Design review of the part built by this model. Coordinates are the model's own, in mm. A direction names the side the tool comes from. Give positions to 0.01 mm unless a question says otherwise; leave off trailing zeros. Loops run counter-clockwise (first coordinate to the right, second up) from the corner with the lowest first, then second, coordinate; pieces in that order, holes last. Notation, with made-up numbers: M -20.75,20 L 35.25,20 A12 cw 35.25,40 Z; hole C 4.25,50 d8. An arc over 180 degrees is marked long. Use a Markdown table: item, result. Add a question column.
(1) Add section D-D, the plane y = -13.5. Give the boundary of the cut face in (x, z), then the cut area to 3 significant figures.
(2) Insertion check: pin 1 Ø1.1 at (y, z) = (-14.5, 16.5) entering from +X; pin 2 Ø0.5 at (x, z) = (7, 22) entering from +Y; pin 3 Ø5 at (x, z) = (2.5, 18) entering from -Y. Each pin has a flat end and moves straight along its axis. Give the tip position at first contact, or say it passes through.
(3) Add section B-B, the plane x = 12. Give the boundary of the cut face in (y, z), then the cut area to 3 significant figures.
(4) Draft analysis for pull direction Y (two halves, no side actions). For faces 1 (the face through (9.67, -1.52, 15.21)), 2 (the face through (13.942, -17.028, 14.79)), 3 (the face through (14.3, -14.5, 14.8)), state which applies: pulls with the +Y half, pulls with the -Y half, needs draft (parallel to the pull), parting line crosses it, or undercut.
(5) Add section A-A, the plane z = 22. Give the boundary of the cut face in (x, y), then the cut area to 3 significant figures.
(6) Add section C-C, the plane z = 8.25. Give the boundary of the cut face in (x, y).
(7) For probe 1 along Z at (x, y) = (6.5, -3.75); probe 2 along Y at (x, z) = (10, 9.75); probe 3 along X at (y, z) = (-3.5, 14), list the stretches that pass through material, from the lowest coordinate up.
(8) For faces 4 (the face through (6.5, -11, 15)), 5 (the face through (20, -5, 15)), 6 (the face through (13.5, -11, 15)), 7 (the face through (6.44, -3.94, 23.38)), 8 (the face through (10, -19, 15)), list the 3-axis set-ups (+Z, -Z, +X, -X, +Y, -Y) from which the entire face can be reached by the end or side of a thin tool; tool diameter is ignored.
```python
from build123d import *
from OCP.BRepFilletAPI import BRepFilletAPI_MakeChamfer

# Parameters (mm, degrees)
BOSS_EXTRUDE1_DEPTH = 30
SKETCH2_R           = 1.45
CUT_EXTRUDE1_DEPTH  = 8
SKETCH3_R           = 2.5
CUT_EXTRUDE2_DEPTH  = 41.755367745
CHAMFER1_SIZE       = 3
CHAMFER2_SIZE       = 4
CHAMFER2_SIZE2      = 0.705307923


with BuildPart() as part:
    # Sketch1 → Boss-Extrude1 (new body)
    with BuildSketch(Plane.XY):
        Polygon((0, 0), (20, 0), (20, -8), (13.5, -8), (13.5, -14), (14.3, -14), (14.3, -19), (5.7, -19), (5.7, -14), (6.5, -14), (6.5, -8), (0, -8), align=None)
    extrude(amount=BOSS_EXTRUDE1_DEPTH)

    # Sketch2 → Cut-Extrude1 (cut)
    with BuildSketch(Plane(origin=(0, 0, 0), x_dir=(1, 0, 0), z_dir=(0, 1, 0))):
        with Locations(Location((14, -22, 0), (0, 0, 270))):
            Circle(SKETCH2_R)
        with Locations(Location((6, -22, 0), (0, 0, 270))):
            Circle(SKETCH2_R)
    extrude(amount=-CUT_EXTRUDE1_DEPTH, mode=Mode.SUBTRACT)

    # Sketch3 → Cut-Extrude2 (cut, through all)
    with BuildSketch(Plane.XY.offset(30)):
        with Locations((10, -4)):
            Circle(SKETCH3_R)
    extrude(amount=-CUT_EXTRUDE2_DEPTH, mode=Mode.SUBTRACT)

    # Chamfer1
    chamfer1_edges = [part.edges().sort_by_distance(p)[0] for p in [
        (0, 0, 15),
        (20, 0, 15),
    ]]
    chamfer(chamfer1_edges, length=CHAMFER1_SIZE)

    # Chamfer2: one chamfer whose edges measure the first distance from different faces: ONE call of the kernel's chamfer builder (chamfer() names one face for all edges)
    chamfer2_edges_1 = [part.edges().sort_by_distance(p)[0] for p in [
        (14.3, -19, 15),
    ]]
    chamfer2_side_1 = [part.faces().sort_by_distance(p)[0] for p in [
        (14.3, -16.5, 15),
    ]]
    chamfer2_edges_2 = [part.edges().sort_by_distance(p)[0] for p in [
        (5.7, -19, 15),
    ]]
    chamfer2_side_2 = [part.faces().sort_by_distance(p)[0] for p in [
        (5.7, -16.5, 15),
    ]]
    chamfer2 = BRepFilletAPI_MakeChamfer(part.part.solid().wrapped)
    for e in chamfer2_edges_1:
        chamfer2.Add(CHAMFER2_SIZE, CHAMFER2_SIZE2, e.wrapped, chamfer2_side_1[0].wrapped)  # the first distance lies on this face
    for e in chamfer2_edges_2:
        chamfer2.Add(CHAMFER2_SIZE, CHAMFER2_SIZE2, e.wrapped, chamfer2_side_2[0].wrapped)  # the first distance lies on this face
    add(Compound.cast(chamfer2.Shape()), mode=Mode.REPLACE)


solid = part.part
```
Established:
| question | item | result |
|---|---|---|
| 1 | outline | M 6.5,0 L 13.5,0 L 13.5,30 L 6.5,30 Z |
| 1 | area | 210 mm^2 |
| 2 | pin 1 | x = 14.3 |
| 2 | pin 2 | y = -8 |
| 2 | pin 3 | y = -8 |
| 3 | outline | M -19,0 L -5.5,0 L -5.5,30 L -19,30 Z; M -2.5,0 L 0,0 L 0,30 L -2.5,30 Z |
| 3 | area | 480 mm^2 |
| 4 | face 1 | undercut |
| 4 | face 2 | pulls with the -Y half |
| 4 | face 3 | needs draft |
| 5 | outline | M 0,-8 L 4.55,-8 L 4.55,0 L 3,0 L 0,-3 Z; M 5.7,-15 L 6.41,-19 L 13.59,-19 L 14.3,-15 L 14.3,-14 L 13.5,-14 L 13.5,-8 L 12.55,-8 L 12.55,0 L 7.45,0 L 7.45,-8 L 6.5,-8 L 6.5,-14 L 5.7,-14 Z; M 15.45,-8 L 20,-8 L 20,-3 L 17,0 L 15.45,0 Z; hole C 10,-4 d5 |
| 5 | area | 167 mm^2 |
| 6 | outline | M 0,-8 L 6.5,-8 L 6.5,-14 L 5.7,-14 L 5.7,-15 L 6.41,-19 L 13.59,-19 L 14.3,-15 L 14.3,-14 L 13.5,-14 L 13.5,-8 L 20,-8 L 20,-3 L 17,0 L 3,0 L 0,-3 Z; hole C 10,-4 d5 |
| 7 | probe 1 | 0 to 20.64, 23.36 to 30 |
| 7 | probe 2 | -19 to -6.5, -1.5 to 0 |
| 7 | probe 3 | 0 to 7.55, 12.45 to 20 |
| 8 | face 4 | +Z, -Z, -X |
| 8 | face 5 | +Z, -Z, +X, +Y, -Y |
| 8 | face 6 | +Z, -Z, +X |
| 8 | face 7 | +Y |
| 8 | face 8 | +Z, -Z, +X, -X, -Y |
